Build history of the part. All positions in model axes, mm. A direction names the side the tool comes from. Give positions to 0.01 mm unless a question says otherwise; leave off trailing zeros. Order: outer loops, then holes, each group sorted by start corner. A loop starts at its lowest first (then second) coordinate and runs counter-clockwise, first axis right, second up. Notation, with made-up numbers: (-26, 8) - (25, 8) arc R29 cw to (25, 45) - close; hole circle Ø5 at (59.5, 37). An arc over 180 degrees is marked (long way). Answer in a Markdown table with one row per item.
```python
from build123d import *

# Parameters (mm, degrees)
BOSS_EXTRUDE1_DEPTH  = 1
M6_CLEARANCE_HOLE1_D = 6.6
SKETCH8_W            = 41.5
SKETCH8_H            = 838.415827604
CUT_EXTRUDE1_DEPTH   = 10
EDGE_FLANGE1_DEPTH   = 690.012501954
FILLET1_R            = 3
M6_CLEARANCE_HOLE2_D = 6.6


# Sheet-metal steps are written as plain solids
with BuildPart() as part:
    # Sketch1 → Boss-Extrude1 (new body)
    with BuildSketch(Plane(origin=(0, 0, 0), x_dir=(1, 0, 0), z_dir=(0, 1, 0))):
        Polygon((-364, -346.881188119), (-364, -385), (364, -385), (364, -346.881188119), (404, -346.881188119), (404, 346.881188119), (364, 346.881188119), (364, 385), (-364, 385), (-364, 346.881188119), (-404, 346.881188119), (-404, -346.881188119), align=None)
    extrude(amount=BOSS_EXTRUDE1_DEPTH)

    # M6 Clearance Hole1 (through all)
    with Locations(Plane(origin=(0, 1, 0), x_dir=(1, 0, 0), z_dir=(0, 1, 0))):
        with Locations((-214, -367.5), (-385, -196.881188119), (-385, 196.881188119), (-214, 367.5), (214, 367.5), (214, -367.5), (385, -286.881188119), (385, -86.881188119)):
            Hole(M6_CLEARANCE_HOLE1_D / 2)

    # Sketch8 → Cut-Extrude1 (cut)
    with BuildSketch(Plane(origin=(0, 1, 0), x_dir=(1, 0, 0), z_dir=(0, 1, 0))):
        with Locations((383.25, -15.625663738)):
            Rectangle(SKETCH8_W, SKETCH8_H)
    extrude(amount=-CUT_EXTRUDE1_DEPTH, mode=Mode.SUBTRACT)

    # Edge-Flange1 section (across the edge) → Edge-Flange1 (add)
    with BuildSketch(Plane(origin=(363.5, 0, -345), x_dir=(-1, 0, 0), z_dir=(0, 0, 1))):
        with BuildLine():
            Line((-1, 1), (-1, 35))
            Line((-1, 35), (0, 35))
            Line((0, 35), (0, 1))
            ThreePointArc((0, 1), (0.292893219, 0.292893219), (1, 0))
            Line((1, 0), (1, -1))
            ThreePointArc((1, -1), (-0.414213562, -0.414213562), (-1, 1))
        make_face()
    extrude(amount=EDGE_FLANGE1_DEPTH)

    # Fillet1
    fillet1_edges = [part.edges().sort_by_distance(p)[0] for p in [
        (364, -35, -345),
        (364, -35, 345.012501954),
        (-364, 0.5, 385),
        (-364, 0.5, 346.881188119),
        (-404, 0.5, 346.881188119),
        (-404, 0.5, -346.881188119),
        (-364, 0.5, -346.881188119),
        (-364, 0.5, -385),
        (362.5, 0.5, -385),
        (362.5, 0.5, 385),
    ]]
    fillet(fillet1_edges, radius=FILLET1_R)

    # M6 Clearance Hole2 (through all)
    with Locations(Plane(origin=(364.5, 0, 0), x_dir=(0, 0, -1), z_dir=(1, 0, 0))):
        with Locations((-225, -20), (225, -20)):
            Hole(M6_CLEARANCE_HOLE2_D / 2)


solid = part.part
```
1. Drop flat-ended pins along their axis: P1, Ø0.5, axis at y = 0.5, z = 368.5, coming from the -X side; P2, Ø0.8, axis at x = -384.5, y = 0.5, coming from the +Z side; P3, Ø10.5, axis at x = 214, z = -367.5, coming from the -Y side. Give the stop position or say it passes through.
Check result:
| item | result |
|---|---|
| P1 | stops at x = -364 |
| P2 | stops at z = 346.88 |
| P3 | stops at y = 0 |
2. Probe line 1 (Z direction, x = -385, y = 0.4); line 2 (Z direction, x = -214, y = 0.7); line 3 (X direction, y = 0.2, z = 367.5). List the from-to ranges inside material, lowest first.
Check result:
| item | result |
|---|---|
| line 1 | z = -346.88 to -200.18, -193.58 to 193.58, 200.18 to 346.88 |
| line 2 | z = -385 to -370.8, -364.2 to 364.2, 370.8 to 385 |
| line 3 | x = -364 to -217.3, -210.7 to 210.7, 217.3 to 362.5 |
3. Cut at B-B on x = -233.5. Write the cut outline in (y, z).
Check result:
| item | result |
|---|---|
| outline | (0, -385) - (1, -385) - (1, 385) - (0, 385) - close |
4. Which spindle directions (+Z, -Z, +X, -X, +Y, -Y) get a long thin tool onto all of the face, cutting with end or side? Do faces 1 (the face through (-26, 0, -5)), 2 (the face through (-26, 1, -5)). Say none if no direction does.
Check result:
| item | result |
|---|---|
| face 1 | +Z, -Z, -X, -Y |
| face 2 | +Z, -Z, +X, -X, +Y |
5. Cut at A-A on z = 169. Write the cut outline in (x, y), and give its area (3 significant figures).
Check result:
| item | result |
|---|---|
| outline | (-404, 0) - (362.5, 0) arc R1 cw to (363.5, -1) - (363.5, -35) - (364.5, -35) - (364.5, -1) arc R2 ccw to (362.5, 1) - (-404, 1) - close |
| area | 803 mm² |
